from build123d import *

# Parameters (mm, degrees)
F0_W     = 63.5
F0_H     = 63.5
F0_W_2   = 57.5
F0_H_2   = 57.5
F1_DEPTH = 290
F2_R     = 8.791749
F3_DEPTH = 25


with BuildPart() as f1:
    # F0 (on Top) → F1 (new body)
    with BuildSketch(Plane.XY):
        with Locations((2.03071, 3.669284)):
            Rectangle(F0_W, F0_H)
        with Locations((2.03071, 3.669284)):
            Rectangle(F0_W_2, F0_H_2, mode=Mode.SUBTRACT)
    extrude(amount=F1_DEPTH)

    # F2 (on face) → F3 (cut)
    with BuildSketch(Plane.YZ.offset(33.78071)):
        with Locations((3.669284, 150)):
            Circle(F2_R)
    extrude(amount=-F3_DEPTH, mode=Mode.SUBTRACT)


solid = f1.part
The model under review builds one solid part; all positions refer to its coordinate system, in mm. A direction names the side the tool comes from. Round coordinates to 2 decimals unless told otherwise and drop trailing zeros. Loops run counter-clockwise (first coordinate to the right, second up) from the corner with the lowest first, then second, coordinate; pieces in that order, holes last. Notation, with made-up numbers: (49.25, 31) -> (59.25, 31) arc R27 cw to (59.25, 56) -> close; hole circle Ø10 at (30, 21.25). An arc over 180 degrees is marked (long way). Answer as CSV lines item,"result".
1) Add section C-C on x = 2.5. Write out the cut boundary in (y, z).
Geometry results:
outline,"(-28.08, 0) -> (-25.08, 0) -> (-25.08, 290) -> (-28.08, 290) -> close; (32.42, 0) -> (35.42, 0) -> (35.42, 290) -> (32.42, 290) -> close"
2) Add section A-A on y = -15.5. Write out the cut boundary in (x, z), plus the area to 3 significant figures.
Geometry results:
outline,"(-29.72, 0) -> (-26.72, 0) -> (-26.72, 290) -> (-29.72, 290) -> close; (30.78, 0) -> (33.78, 0) -> (33.78, 290) -> (30.78, 290) -> close"
area,"1,740 mm²"
3) Draft analysis for pull direction Y (two halves, no side actions). For faces 1 (the face through (2, 35.419, 143)), 2 (the face through (2, -28.081, 143)), 3 (the face through (2, -25.081, 143)), state which applies: pulls with the +Y half, pulls with the -Y half, needs draft (parallel to the pull), parting line crosses it, or undercut.
Geometry results:
face 1,"pulls with the +Y half"
face 2,"pulls with the -Y half"
face 3,"undercut"
4) Tool access review of faces 4 (the face through (-26.719, 3, 143)), 5 (the face through (0, -27, 290)), 6 (the face through (32.3, 1.76, 141.42)): name each direction out of +Z, -Z, +X, -X, +Y, -Y from which nothing blocks a thin tool from reaching the whole face with its end or side.
Geometry results:
face 4,"+Z, -Z"
face 5,"+Z, +X, -X, +Y, -Y"
face 6,"+X"
5) Add section B-B on z = 109.5. Write out the cut boundary in (x, y).
Geometry results:
outline,"(-29.72, -28.08) -> (33.78, -28.08) -> (33.78, 35.42) -> (-29.72, 35.42) -> close; hole (-26.72, -25.08) -> (30.78, -25.08) -> (30.78, 32.42) -> (-26.72, 32.42) -> close"
6) Add section D-D on z = 150. Write out the cut boundary in (x, y).
Geometry results:
outline,"(-29.72, -28.08) -> (33.78, -28.08) -> (33.78, -5.12) -> (30.78, -5.12) -> (30.78, -25.08) -> (-26.72, -25.08) -> (-26.72, 32.42) -> (30.78, 32.42) -> (30.78, 12.46) -> (33.78, 12.46) -> (33.78, 35.42) -> (-29.72, 35.42) -> close"
7) To check wall thickness, follow line 1 along X through (y, z) = (-14.5, 74); line 2 along Y through (x, z) = (1.5, 122). State the ranges of each line that lie inside material, in increasing order. Write a range as from..to.
Geometry results:
line 1,"x = -29.72..-26.72, 30.78..33.78"
line 2,"y = -28.08..-25.08, 32.42..35.42"
8) For P1, Ø5, axis at x = -22, y = -20, coming from the +Z side, flat-tipped, find the tip position at first contact; note if it passes through.
Geometry results:
P1,"passes through"
